Study the drawing (mm; zero at the part's minimum x, y, z) and answer. A direction names the side the tool comes from. Coordinates: 2 decimals unless noted, no trailing zeros. Order: outer loops, then holes, each group sorted by start corner. A loop starts at its lowest first (then second) coordinate and runs counter-clockwise, first axis right, second up. Notation, with made-up numbers: (65, -17) -> (117, -17) arc R29 cw to (117, 6) -> close; hole circle Ø8 at (30, -37). An arc over 180 degrees is marked (long way). Write each question's results on one line, items separated by ' | '. Start each with the question number.
(1) Given pin 1 (6 mm diameter, centred on y = 33, z = 6.5, fed in from +X); pin 2 (3 mm diameter, centred on x = 31.39, y = 15, fed in from +Z); pin 3 (5 mm diameter, centred on x = 10.61, y = 27, fed in from -Z); pin 4 (8 mm diameter, centred on y = 27.5, z = 12, fed in from -X), each flat-ended and moving along its own axis, determine where each tip first touches the part or whether it passes through.
(2) The part is cut by section A-A, the plane x = 21. Give the vertices of the cut face in (y, z), then the cut area to 3 significant figures.
(3) The part is cut by section D-D, the plane z = 12.5. Give the vertices of the cut face in (x, y).
(4) The part is cut by section B-B, the plane y = 9. Give the vertices of the cut face in (x, z).
(5) Determine the mould class of the marked faces 4, 5 and 6 for opening direction X: +X half, -X half, draft (parallel to the pull), parting line (faces both ways), or undercut.
(6) The part is cut by section C-C, the plane x = 10. Give the vertices of the cut face in (y, z) (1 decimal), then the cut area to 3 significant figures.
(7) A tool of negligible diameter and unlimited length cuts with its end or side. For the marked faces 1, 2 and 3, from which of +Z, -Z, +X, -X, +Y, -Y can it reach the whole face along a straight path? Write none if from no direction.
(8) Straight lines are drawn through the part: L1, parallel to Y at x = 21, z = 4.75; L2, parallel to Y at x = 21, z = 1.3; L3, parallel to X at y = 15.5, z = 9 (1 decimal). For each, find the intervals that lie inside material, in ascending order.
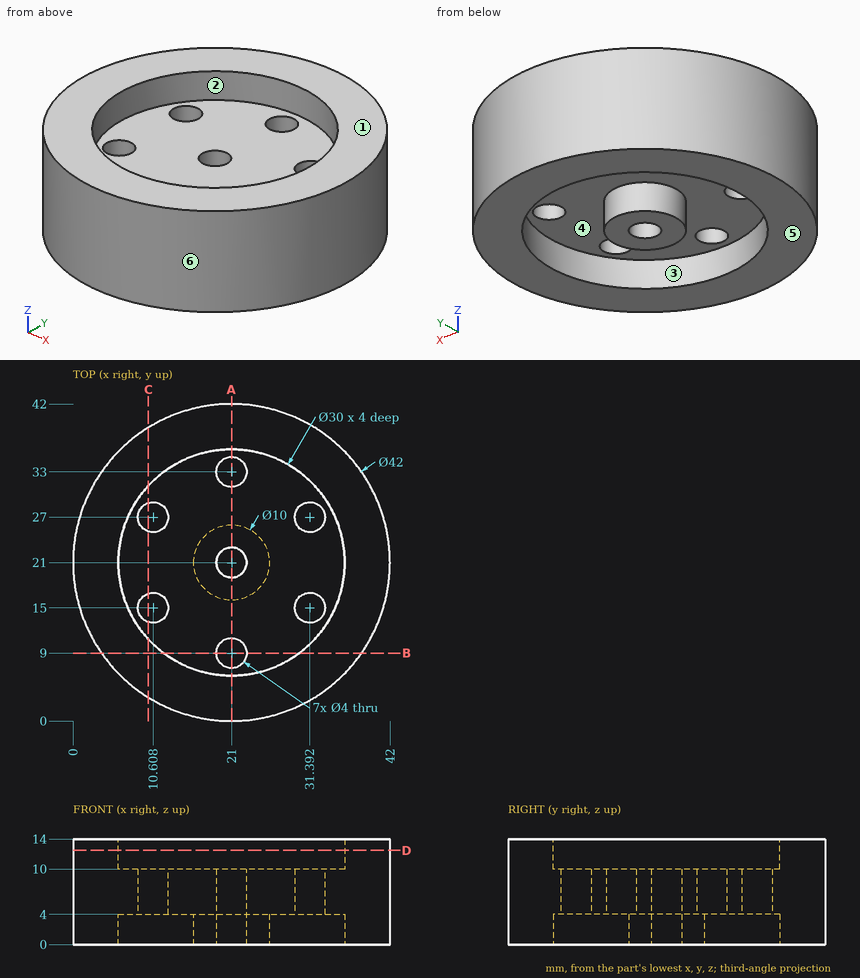
Established:
1) pin 1: stops at x = 39.97 | pin 2: passes through | pin 3: stops at z = 4 | pin 4: stops at x = 0.15
2) outline: (0, 0) -> (6, 0) -> (6, 4) -> (7, 4) -> (7, 10) -> (6, 10) -> (6, 14) -> (0, 14) -> close; (11, 4) -> (16, 4) -> (16, 0) -> (19, 0) -> (19, 10) -> (11, 10) -> close; (23, 0) -> (26, 0) -> (26, 4) -> (31, 4) -> (31, 10) -> (23, 10) -> close; (35, 4) -> (36, 4) -> (36, 0) -> (42, 0) -> (42, 14) -> (36, 14) -> (36, 10) -> (35, 10) -> close | area: 300 mm^2
3) outline: circle Ø42 at (21, 21); hole circle Ø30 at (21, 21)
4) outline: (3.77, 0) -> (12, 0) -> (12, 4) -> (19, 4) -> (19, 10) -> (12, 10) -> (12, 14) -> (3.77, 14) -> close; (23, 4) -> (30, 4) -> (30, 0) -> (38.23, 0) -> (38.23, 14) -> (30, 14) -> (30, 10) -> (23, 10) -> close
5) face 4: undercut | face 5: draft | face 6: parting line
6) outline: (3.1, 0) -> (10.8, 0) -> (10.8, 4) -> (13.1, 4) -> (13.1, 10) -> (10.8, 10) -> (10.8, 14) -> (3.1, 14) -> close; (16.9, 4) -> (25.1, 4) -> (25.1, 10) -> (16.9, 10) -> close; (28.9, 4) -> (31.2, 4) -> (31.2, 0) -> (38.9, 0) -> (38.9, 14) -> (31.2, 14) -> (31.2, 10) -> (28.9, 10) -> close | area: 292 mm^2
7) face 1: +Z, +X, -X, +Y, -Y | face 2: +Z | face 3: -Z
8) L1: y = 0 to 7, 11 to 19, 23 to 31, 35 to 42 | L2: y = 0 to 6, 16 to 19, 23 to 26, 36 to 42 | L3: x = 0.7 to 8.7, 12.5 to 29.5, 33.3 to 41.3
